```python
from build123d import *

# Parameters (mm, degrees)
SKETCH1_R           = 20.356349186
SKETCH1_R_2         = 1.6
BOSS_EXTRUDE1_DEPTH = 8
CHAMFER1_SIZE       = 0.4


with BuildPart() as part:
    # Sketch1 → Boss-Extrude1 (new body)
    with BuildSketch(Plane(origin=(0, 0, 0), x_dir=(1, 0, 0), z_dir=(0, 1, 0))):
        Circle(SKETCH1_R)
        Circle(SKETCH1_R_2, mode=Mode.SUBTRACT)
        with Locations((-11, 11)):
            Circle(SKETCH1_R_2, mode=Mode.SUBTRACT)
        with Locations((11, 11)):
            Circle(SKETCH1_R_2, mode=Mode.SUBTRACT)
        with Locations((11, -11)):
            Circle(SKETCH1_R_2, mode=Mode.SUBTRACT)
        with Locations((-11, -11)):
            Circle(SKETCH1_R_2, mode=Mode.SUBTRACT)
    extrude(amount=BOSS_EXTRUDE1_DEPTH)

    # Chamfer1
    chamfer1_edges = [part.edges().sort_by_distance(p)[0] for p in [
        (9.4, 0, -11),
        (9.4, 8, -11),
        (9.4, 0, 11),
        (9.4, 8, 11),
        (-20.356349186, 0, 0),
        (-12.6, 0, 11),
        (-12.6, 8, 11),
        (-20.356349186, 8, 0),
        (-1.6, 0, 0),
        (-1.6, 8, 0),
        (-12.6, 0, -11),
        (-12.6, 8, -11),
    ]]
    chamfer(chamfer1_edges, length=CHAMFER1_SIZE)


solid = part.part
```
Can you work these out from the model? Positions are in its coordinate system, mm. Round coordinates to 2 decimals unless told otherwise and drop trailing zeros. Loops run counter-clockwise (first coordinate to the right, second up) from the corner with the lowest first, then second, coordinate; pieces in that order, holes last. Notation, with made-up numbers: M 4.5,-11 L 39.5,-11 A23 cw 39.5,2 Z; hole C 80,84.25 d1. An arc over 180 degrees is marked long. Answer as a JSON object with one key per item and string values. Group by question number.
Q1. Imagine slicing it at A-A, the plane z = 0. Please give me the cut outline in (x, y), then the cut area to 3 significant figures.
Q2. Will these pins go through, and if not, where does the flat tip stop? pin 1 (3.5 mm diameter, centred on x = -11, z = 11, fed in from -Y); pin 2 (8 mm diameter, centred on x = 14.5, z = 7, fed in from -Y); pin 3 (3 mm diameter, centred on x = 14, y = 7, fed in from -Z); pin 4 (3.5 mm diameter, centred on x = 0, z = 0, fed in from +Y).
Q3. We'd pull the mould along X, two halves only. Please class faces 1 (the cylindrical face through (-4.413, 3.95, 19.872)), 2 (the flat face through (4, 8, 0)), 3 (the cylindrical face through (9.4, 3.95, 10.93)): +X half, -X half, draft (parallel to the pull), parting line (faces both ways), or undercut.
Q4. Imagine slicing it at C-C, the plane y = 6. Please give me the cut outline in (x, z), then the cut area to 3 significant figures.
Q5. Imagine slicing it at D-D, the plane z = -11. Count the separate pieces of the cut face and the enclosed holes in it, then the cut area to 3 significant figures.
Q6. Please list where these lines run through material, in increasing order: L1, parallel to X at y = 2, z = 0; L2, parallel to X at y = 2.25, z = 11.
Q7. Imagine slicing it at B-B, the plane x = 0. Please give me the cut outline in (y, z).
Findings:
{
 "1": {"outline": "M -20.36,0.4 L -19.96,0 L -2,0 L -1.6,0.4 L -1.6,7.6 L -2,8 L -19.96,8 L -20.36,7.6 Z; M 1.6,0.4 L 2,0 L 19.96,0 L 20.36,0.4 L 20.36,7.6 L 19.96,8 L 2,8 L 1.6,7.6 Z", "area": "299 mm2"},
 "2": {"pin 1": "stops at y = 0.25", "pin 2": "stops at y = 0", "pin 3": "stops at z = -16.07", "pin 4": "stops at y = 7.75"},
 "3": {"face 1": "parting line", "face 2": "draft", "face 3": "undercut"},
 "4": {"outline": "C 0,0 d40.71; hole C -11,-11 d3.2; hole C -11,11 d3.2; hole C 0,0 d3.2; hole C 11,-11 d3.2; hole C 11,11 d3.2", "area": "1,260 mm2"},
 "5": {"separate pieces": "3", "enclosed holes": "0", "area": "222 mm2"},
 "6": {"L1": "x = -20.36 to -1.6, 1.6 to 20.36", "L2": "x = -17.13 to -12.6, -9.4 to 9.4, 12.6 to 17.13"},
 "7": {"outline": "M 0,-19.96 L 0.4,-20.36 L 7.6,-20.36 L 8,-19.96 L 8,-2 L 7.6,-1.6 L 0.4,-1.6 L 0,-2 Z; M 0,2 L 0.4,1.6 L 7.6,1.6 L 8,2 L 8,19.96 L 7.6,20.36 L 0.4,20.36 L 0,19.96 Z"}
}
